from build123d import *

# Parameters (mm, degrees)
SKETCH1_W           = 965
SKETCH1_H           = 508
BOSS_EXTRUDE1_DEPTH = 100
SKETCH5_R           = 20
CUT_EXTRUDE1_DEPTH  = 50


with BuildPart() as part:
    # Sketch1 → Boss-Extrude1 (new body)
    with BuildSketch(Plane(origin=(0, 0, 0), x_dir=(1, 0, 0), z_dir=(0, 1, 0))):
        Rectangle(SKETCH1_W, SKETCH1_H)
    extrude(amount=BOSS_EXTRUDE1_DEPTH)

    # Sketch5 → Cut-Extrude1 (cut)
    with BuildSketch(Plane.XZ):
        with Locations(Location((254, 204, 0), (0, 0, 270))):
            Circle(SKETCH5_R)
        with Locations(Location((254, -204, 0), (0, 0, 270))):
            Circle(SKETCH5_R)
    cut_extrude1 = extrude(amount=-CUT_EXTRUDE1_DEPTH, mode=Mode.SUBTRACT)

    # Mirror1: Cut-Extrude1 across plane
    add(cut_extrude1.mirror(Plane(origin=(0, 0, 0), x_dir=(0, 0, 1), z_dir=(1, 0, 0))), mode=Mode.SUBTRACT)


solid = part.part
Work out the finished part from the listing and answer in its coordinate system (mm). A direction names the side the tool comes from. Round coordinates to 2 decimals unless told otherwise and drop trailing zeros. Loops run counter-clockwise (first coordinate to the right, second up) from the corner with the lowest first, then second, coordinate; pieces in that order, holes last. Notation, with made-up numbers: (8.5, 82) - (50.5, 82) arc R24 ccw to (50.5, 95) - close; hole circle Ø5 at (29.5, 41). An arc over 180 degrees is marked (long way). One line per item, written item: value.
Q1. For faces 5 (the flat face through (-7, 100, -4)), 6 (the cylindrical face through (-267.52, 24.65, 218.74)), determine the directions among +Z, -Z, +X, -X, +Y, -Y from which every point of the face is accessible in a straight line to the end or side of a thin tool.
Check values:
face 5: +Z, -Z, +X, -X, +Y
face 6: -Y
Q2. Find section B-B on x = 254. Give the vertices of the cut face in (y, z).
Check values:
outline: (0, -254) - (100, -254) - (100, 254) - (0, 254) - (0, 224) - (50, 224) - (50, 184) - (0, 184) - (0, -184) - (50, -184) - (50, -224) - (0, -224) - close
Q3. This flat-tipped pin is pushed along its axis until it touches: pin 1 Ø12 at (x, z) = (252.5, 210.5) entering from -Y. Where does it stop, or does it pass through?
Check values:
pin 1: y = 50
Q4. Straight lines are drawn through the part: probe 1 along X at (y, z) = (15.5, -204); probe 2 along Z at (x, y) = (-254, 37); probe 3 along X at (y, z) = (10, 221). For each, find the intervals that lie inside material, in ascending order.
Check values:
probe 1: -482.5 to -274, -234 to 234, 274 to 482.5
probe 2: -254 to -224, -184 to 184, 224 to 254
probe 3: -482.5 to -264.54, -243.46 to 243.46, 264.54 to 482.5
Q5. The mould has two halves that part along X. Classify faces 1 (the flat face through (254, 50, 204)), 2 (the flat face through (-7, 0, -4)), 3 (the flat face through (482.5, 49, 4)), 4 (the flat face through (-482.5, 49, 4)): +X half, -X half, draft (parallel to the pull), parting line (faces both ways), or undercut.
Check values:
face 1: undercut
face 2: draft
face 3: +X half
face 4: -X half
Q6. Find section A-A on z = 204. Give the vertices of the cut face in (x, y).
Check values:
outline: (-482.5, 0) - (-274, 0) - (-274, 50) - (-234, 50) - (-234, 0) - (234, 0) - (234, 50) - (274, 50) - (274, 0) - (482.5, 0) - (482.5, 100) - (-482.5, 100) - close
